The model under review builds one solid part; all positions refer to its coordinate system, in mm. A direction names the side the tool comes from. Coordinates: 2 decimals unless noted, no trailing zeros. Loops run counter-clockwise (first coordinate to the right, second up) from the corner with the lowest first, then second, coordinate; pieces in that order, holes last. Notation, with made-up numbers: (27, -25) - (80, -25) arc R13 cw to (80, -8) - close; hole circle Ø7 at (-35, -19). An arc over 180 degrees is marked (long way). Use a Markdown table: item, result. Add a question column.
1) The part is to be moulded in two halves that separate along X. For faces 3 (the flat face through (-0.1, -4.3, 0)), 4 (the cylindrical face through (6.22, 2.05, 1.48)), say which applies: pulls with the +X half, pulls with the -X half, needs draft (parallel to the pull), parting line crosses it, or undercut.
2) For faces 1 (the flat face through (-0.1, -4.3, 3)), 2 (the flat face through (-5.2, 0, 1)), list the 3-axis set-ups (+Z, -Z, +X, -X, +Y, -Y) from which the entire face can be reached by the end or side of a thin tool; tool diameter is ignored.
3) Add section B-B, the plane x = 0. Give the boundary of the cut face in (y, z).
4) To check wall thickness, follow L1, parallel to Y at x = 0, z = 1.8; L2, parallel to Y at x = 1.75, z = 1.3; L3, parallel to Y at x = -6.25, z = 1.1. State the ranges of each line that lie inside material, in increasing order. Write a range as [from, to].
5) Add section D-D, the plane y = 3. Give the boundary of the cut face in (x, z), and give its area (3 significant figures).
6) Add section A-A, the plane z = 0.75. Give the boundary of the cut face in (x, y).
```python
from build123d import *

# Parameters (mm, degrees)
SKETCH_1_R          = 10
EXTRUDE_1_DEPTH     = 3
SKETCH_2_R          = 4
CUT_EXTRUDE_1_DEPTH = 4


with BuildPart() as part:
    # 草圖1 → 填料-伸長1 (new body)
    with BuildSketch(Plane.XY):
        Circle(SKETCH_1_R)
    extrude(amount=EXTRUDE_1_DEPTH)

    # 草圖2 → 除料-伸長1 (cut)
    with BuildSketch(Plane.XY):
        Circle(SKETCH_2_R)
        with BuildLine():
            Line((-1.05, 7.2), (1.05, 7.2))
            ThreePointArc((1.05, 7.2), (2.05, 6.2), (1.05, 5.2))
            Line((1.05, 5.2), (-1.05, 5.2))
            ThreePointArc((-1.05, 5.2), (-2.05, 6.2), (-1.05, 7.2))
        make_face()
        with BuildLine():
            Line((-5.2, 1.05), (-5.2, -1.05))
            ThreePointArc((-5.2, -1.05), (-6.2, -2.05), (-7.2, -1.05))
            Line((-7.2, -1.05), (-7.2, 1.05))
            ThreePointArc((-7.2, 1.05), (-6.2, 2.05), (-5.2, 1.05))
        make_face()
        with BuildLine():
            Line((5.2, 1.05), (5.2, -1.05))
            ThreePointArc((5.2, -1.05), (6.2, -2.05), (7.2, -1.05))
            Line((7.2, -1.05), (7.2, 1.05))
            ThreePointArc((7.2, 1.05), (6.2, 2.05), (5.2, 1.05))
        make_face()
        with BuildLine():
            Line((-1.05, -7.2), (1.05, -7.2))
            ThreePointArc((1.05, -7.2), (2.05, -6.2), (1.05, -5.2))
            Line((1.05, -5.2), (-1.05, -5.2))
            ThreePointArc((-1.05, -5.2), (-2.05, -6.2), (-1.05, -7.2))
        make_face()
    extrude(amount=CUT_EXTRUDE_1_DEPTH, mode=Mode.SUBTRACT)


solid = part.part
```
From the geometry:
| question | item | result |
|---|---|---|
| 1 | face 3 | needs draft |
| 1 | face 4 | undercut |
| 2 | face 1 | +Z, +X, -X, +Y, -Y |
| 2 | face 2 | +Z, -Z |
| 3 | outline | (-10, 0) - (-7.2, 0) - (-7.2, 3) - (-10, 3) - close; (-5.2, 0) - (-4, 0) - (-4, 3) - (-5.2, 3) - close; (4, 0) - (5.2, 0) - (5.2, 3) - (4, 3) - close; (7.2, 0) - (10, 0) - (10, 3) - (7.2, 3) - close |
| 4 | L1 | y = [-10, -7.2], [-5.2, -4], [4, 5.2], [7.2, 10] |
| 4 | L2 | y = [-9.85, -6.91], [-5.49, -3.6], [3.6, 5.49], [6.91, 9.85] |
| 4 | L3 | y = [-7.81, -2.05], [2.05, 7.81] |
| 5 | outline | (-9.54, 0) - (-2.65, 0) - (-2.65, 3) - (-9.54, 3) - close; (2.65, 0) - (9.54, 0) - (9.54, 3) - (2.65, 3) - close |
| 5 | area | 41.4 mm^2 |
| 6 | outline | circle Ø20 at (0, 0); hole (-7.2, -1.05) arc R1 ccw to (-5.2, -1.05) - (-5.2, 1.05) arc R1 ccw to (-7.2, 1.05) - close; hole circle Ø8 at (0, 0); hole (-1.05, -7.2) - (1.05, -7.2) arc R1 ccw to (1.05, -5.2) - (-1.05, -5.2) arc R1 ccw to start; hole (-1.05, 5.2) - (1.05, 5.2) arc R1 ccw to (1.05, 7.2) - (-1.05, 7.2) arc R1 ccw to start; hole (5.2, -1.05) arc R1 ccw to (7.2, -1.05) - (7.2, 1.05) arc R1 ccw to (5.2, 1.05) - close |
